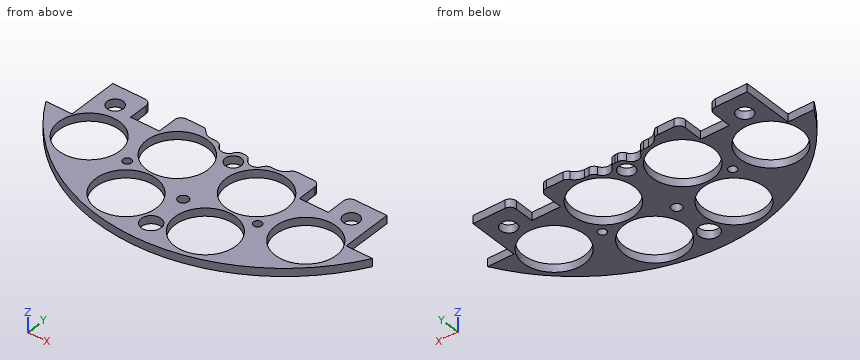
from build123d import *

# Parameters (mm, degrees)
SKETCH1_R                = 1.651
BOSS_EXTRUDE2_DEPTH      = 3.175
SKETCH2_R                = 1.143
CUT_EXTRUDE1_DEPTH       = 4.175
SKETCH3_R                = 12.1285
CUT_EXTRUDE2_DEPTH       = 4.175
SKETCH4_W                = 28.562713242
SKETCH4_H                = 11.677503754
BOSS_EXTRUDE3_DEPTH      = 3.175
SKETCH5_W                = 216.7214489
SKETCH5_H                = 130.569220634
CUT_EXTRUDE4_DEPTH       = 4.175
SKETCH11_R               = 3.937
CUT_EXTRUDE11_DEPTH      = 4.175
SKETCH12_W               = 11.43
SKETCH12_H               = 10.16
CUT_EXTRUDE12_DEPTH      = 4.175
SKETCH16_R               = 12.192
CUT_EXTRUDE16_DEPTH      = 21.59
SKETCH57_R               = 1.651
CUT_EXTRUDE57_DEPTH      = 58.674
SKETCH58_R               = 3.175
CUT_EXTRUDE58_DEPTH      = 103.378
CUT_EXTRUDE58_DEPTH_BACK = 48.768
CUT_EXTRUDE15_DEPTH      = 21.59
FILLET1_R                = 2.54
SKETCH59_R               = 2.032
CUT_EXTRUDE59_DEPTH      = 11.938


with BuildPart() as part:
    # Sketch1 → Boss-Extrude2 (new body)
    with BuildSketch(Plane.XY):
        with BuildLine():
            Line((-64.964441474, 37.338), (-54.550441474, 37.338))
            Line((-54.550441474, 37.338), (-54.550441474, -37.338))
            Line((-54.550441474, -37.338), (-64.964441474, -37.338))
            ThreePointArc((-64.964441474, -37.338), (0, -74.93), (64.964441474, -37.338))
            Line((64.964441474, -37.338), (54.550441474, -37.338))
            Line((54.550441474, -37.338), (54.550441474, 37.338))
            Line((54.550441474, 37.338), (64.964441474, 37.338))
            ThreePointArc((64.964441474, 37.338), (0, 74.93), (-64.964441474, 37.338))
        make_face()
        with Locations((-46.482, 11.049)):
            Circle(SKETCH1_R, mode=Mode.SUBTRACT)
        with Locations((-21.083270032, 10.795)):
            Circle(SKETCH1_R, mode=Mode.SUBTRACT)
        with Locations((-21.083270032, -10.795)):
            Circle(SKETCH1_R, mode=Mode.SUBTRACT)
        with Locations((-46.482, -11.049)):
            Circle(SKETCH1_R, mode=Mode.SUBTRACT)
        with Locations((46.482, -11.049)):
            Circle(SKETCH1_R, mode=Mode.SUBTRACT)
        with Locations((21.083270032, -10.795)):
            Circle(SKETCH1_R, mode=Mode.SUBTRACT)
        with Locations((21.083270032, 10.795)):
            Circle(SKETCH1_R, mode=Mode.SUBTRACT)
        with Locations((46.482, 11.049)):
            Circle(SKETCH1_R, mode=Mode.SUBTRACT)
    extrude(amount=BOSS_EXTRUDE2_DEPTH)

    # Sketch2 → Cut-Extrude1 (cut, through all)
    with BuildSketch(Plane.XY.offset(3.175)):
        with Locations((-6.731, 62.23)):
            Circle(SKETCH2_R)
        with Locations((6.731, 62.23)):
            Circle(SKETCH2_R)
    extrude(amount=-CUT_EXTRUDE1_DEPTH, mode=Mode.SUBTRACT)

    # Sketch3 → Cut-Extrude2 (cut, through all)
    with BuildSketch(Plane(origin=(0, 0, 0), x_dir=(-1, 0, 0), z_dir=(0, 0, -1))):
        with Locations((-15.777608989, -58.882838371)):
            Circle(SKETCH3_R)
        with Locations((15.777608989, -58.882838371)):
            Circle(SKETCH3_R)
        with Locations((-43.105229381, -43.105229381)):
            Circle(SKETCH3_R)
        with Locations((-43.105229381, 43.105229381)):
            Circle(SKETCH3_R)
        with Locations((43.105229381, 43.105229381)):
            Circle(SKETCH3_R)
        with Locations((43.105229381, -43.105229381)):
            Circle(SKETCH3_R)
    extrude(amount=-CUT_EXTRUDE2_DEPTH, mode=Mode.SUBTRACT)

    # Sketch4 → Boss-Extrude3 (add)
    with BuildSketch(Plane(origin=(0, 0, 0), x_dir=(-1, 0, 0), z_dir=(0, 0, -1))):
        with Locations((-1.488809975, 62.152540216)):
            Rectangle(SKETCH4_W, SKETCH4_H)
    extrude(amount=-BOSS_EXTRUDE3_DEPTH)

    # Sketch5 → Cut-Extrude4 (cut, through all)
    with BuildSketch(Plane(origin=(0, 0, 0), x_dir=(-1, 0, 0), z_dir=(0, 0, -1))):
        with Locations((23.316688373, 48.139610317)):
            Rectangle(SKETCH5_W, SKETCH5_H)
    extrude(amount=-CUT_EXTRUDE4_DEPTH, mode=Mode.SUBTRACT)

    # Sketch11 → Cut-Extrude11 (cut, through all)
    with BuildSketch(Plane(origin=(0, 0, 0), x_dir=(-1, 0, 0), z_dir=(0, 0, -1))):
        with Locations((0, -66.045)):
            Circle(SKETCH11_R)
    extrude(amount=-CUT_EXTRUDE11_DEPTH, mode=Mode.SUBTRACT)

    # Sketch12 → Cut-Extrude12 (cut, through all)
    with BuildSketch(Plane(origin=(0, 0, 0), x_dir=(-1, 0, 0), z_dir=(0, 0, -1))):
        with Locations((-33.595441474, -22.225)):
            Rectangle(SKETCH12_W, SKETCH12_H)
        with Locations((33.595441474, -22.225)):
            Rectangle(SKETCH12_W, SKETCH12_H)
    extrude(amount=-CUT_EXTRUDE12_DEPTH, mode=Mode.SUBTRACT)

    # Sketch16 → Cut-Extrude16 (cut)
    with BuildSketch(Plane(origin=(0, 0, 0), x_dir=(-1, 0, 0), z_dir=(0, 0, -1))):
        with Locations((15.777608989, -33.482838371)):
            Circle(SKETCH16_R)
        with Locations((-15.777608989, -33.482838371)):
            Circle(SKETCH16_R)
    extrude(amount=-CUT_EXTRUDE16_DEPTH, mode=Mode.SUBTRACT)

    # Sketch57 → Cut-Extrude57 (cut)
    with BuildSketch(Plane(origin=(0, 0, 0), x_dir=(-1, 0, 0), z_dir=(0, 0, -1))):
        with Locations((-25.937608989, -45.645229381)):
            Circle(SKETCH57_R)
        with Locations((25.937608989, -45.645229381)):
            Circle(SKETCH57_R)
    extrude(amount=-CUT_EXTRUDE57_DEPTH, mode=Mode.SUBTRACT)

    # Sketch58 → Cut-Extrude58 (cut, two sides)
    with BuildSketch(Plane(origin=(30.092005081, 4.08352975, 36.1315), x_dir=(-1, 0, 0), z_dir=(0, 0, -1))) as cut_extrude58_sk:
        with Locations((77.082005081, -29.48352975)):
            Circle(SKETCH58_R)
        with Locations((30.092005081, -29.48352975)):
            Circle(SKETCH58_R)
        with Locations((-16.897994919, -29.48352975)):
            Circle(SKETCH58_R)
    extrude(amount=CUT_EXTRUDE58_DEPTH, mode=Mode.SUBTRACT)
    extrude(cut_extrude58_sk.sketch, amount=-CUT_EXTRUDE58_DEPTH_BACK, mode=Mode.SUBTRACT)

    # Sketch15 → Cut-Extrude15 (cut)
    with BuildSketch(Plane(origin=(0, 0, 0), x_dir=(-1, 0, 0), z_dir=(0, 0, -1))):
        with BuildLine():
            Line((-12.7, -20.24), (-8.888991966, -20.24))
            ThreePointArc((-8.888991966, -20.24), (-5.715, -23.495), (-2.541008034, -20.24))
            Line((-2.541008034, -20.24), (2.541008034, -20.24))
            ThreePointArc((2.541008034, -20.24), (5.715, -23.495), (8.888991966, -20.24))
            Line((8.888991966, -20.24), (12.7, -20.24))
            ThreePointArc((12.7, -20.24), (16.235533906, -11.704466094), (7.7, -15.24))
            Line((7.7, -15.24), (-1.06, -15.24))
            ThreePointArc((-1.06, -15.24), (-4.010609847, -10.6792983), (-9.38, -11.501337137))
            ThreePointArc((-9.38, -11.501337137), (-17.374040774, -13.464234575), (-12.7, -20.24))
        make_face()
    extrude(amount=-CUT_EXTRUDE15_DEPTH, mode=Mode.SUBTRACT)

    # Fillet1
    fillet1_edges = [part.edges().sort_by_distance(p)[0] for p in [
        (39.310441474, -17.145, 1.5875),
        (27.880441474, -17.145, 1.5875),
        (-27.880441474, -17.145, 1.5875),
        (-39.310441474, -17.145, 1.5875),
        (-17.322875188, -17.145, 1.5875),
        (17.322875188, -17.145, 1.5875),
        (-8.888991966, -20.24, 1.5875),
        (-2.541008034, -20.24, 1.5875),
        (2.541008034, -20.24, 1.5875),
        (8.888991966, -20.24, 1.5875),
    ]]
    fillet(fillet1_edges, radius=FILLET1_R)

    # Sketch59 → Cut-Extrude59 (cut)
    with BuildSketch(Plane(origin=(0, 0, 0), x_dir=(-1, 0, 0), z_dir=(0, 0, -1))):
        with Locations((0, -50.165)):
            Circle(SKETCH59_R)
    extrude(amount=-CUT_EXTRUDE59_DEPTH, mode=Mode.SUBTRACT)


solid = part.part
Check sheet for the modelled part. Datum: model origin and axes. Units: mm. Give positions to 0.01 mm unless a question says otherwise; leave off trailing zeros. Loops run counter-clockwise (first coordinate to the right, second up) from the corner with the lowest first, then second, coordinate; pieces in that order, holes last. Notation, with made-up numbers: M 44.25,-19.5 L 80.25,-19.5 A22 cw 80.25,-12.5 Z; hole C -34.5,-37.5 d7. An arc over 180 degrees is marked long. Answer as a JSON object with one key per item and string values. Group by question number.
Q1. Go/stop test with flat-tipped pins: P1, Ø7.5, axis at x = 0, y = -25.4, coming from the -Z side; P2, Ø0.9, axis at x = 11.5, z = 2, coming from the +Y side; P3, Ø1, axis at y = -34, z = 3, coming from the -X side; P4, Ø1, axis at y = -55.5, z = 2, coming from the -X side. Record where each tip stops, or that it passes through.
Q2. Cross-section at A-A on x = -48. Record the cut outline in (y, z) (3 decimals).
Q3. Cross-section at B-B on y = -39.5. Record the cut outline in (x, z) (1 decimal), then the cut area to 3 significant figures.
Q4. Cross-section at C-C on y = -25.4. Give the number of separate pieces and of enclosed holes in the cut face, then the cut area to 3 significant figures.
Q5. Material ranges on line 1 along X through (y, z) = (-46.5, 2.85); line 2 along Y through (x, z) = (2.5, 1.7); line 3 along Y through (x, z) = (-20, 2) (3 decimals), recorded low to high. Write a range as [from, to].
Evaluation:
{
 "1": {"P1": "stops at z = 0", "P2": "stops at y = -20.24", "P3": "stops at x = -54.55", "P4": "stops at x = -50.89"},
 "2": {"outline": "M -57.537,0 L -54.202,0 L -54.202,3.175 L -57.537,3.175 Z; M -32.008,0 L -28.41,0 L -28.41,3.175 L -32.008,3.175 Z; M -22.39,0 L -17.145,0 L -17.145,3.175 L -22.39,3.175 Z"},
 "3": {"outline": "M -63.7,0 L -54.7,0 L -54.7,3.2 L -63.7,3.2 Z; M -31.5,0 L -26.4,0 L -26.4,3.2 L -31.5,3.2 Z; M -5.2,0 L 5.2,0 L 5.2,3.2 L -5.2,3.2 Z; M 26.4,0 L 31.5,0 L 31.5,3.2 L 26.4,3.2 Z; M 54.7,0 L 63.7,0 L 63.7,3.2 L 54.7,3.2 Z", "area": "123 mm2"},
 "4": {"separate pieces": "8", "enclosed holes": "0", "area": "97.4 mm2"},
 "5": {"line 1": "x = [-58.76, -54.75], [-31.46, -27.35], [-24.53, 24.53], [27.35, 31.46], [54.75, 58.76]", "line 2": "y = [-74.89, -69.09], [-63, -27.36], [-23.44, -21.14]", "line 3": "y = [-72.212, -70.253], [-47.513, -44.92], [-22.045, -17.145]"}
}
